```python
from build123d import *

# Parameters (mm, degrees)
SKIZZE1_R                        = 50
SKIZZE1_R_2                      = 20
AUFSATZ_LINEAR_AUSTRAGEN1_DEPTH  = 2.75
F_3_2_3_2_DURCHMESSER_BOHRUNG1_D = 3.2
KREISMUSTER1_COUNT               = 7


with BuildPart() as part:
    # Skizze1 → Aufsatz-Linear austragen1 (new body)
    with BuildSketch(Plane.XY):
        Circle(SKIZZE1_R)
        Circle(SKIZZE1_R_2, mode=Mode.SUBTRACT)
    extrude(amount=AUFSATZ_LINEAR_AUSTRAGEN1_DEPTH)

    # Ø3.2 (3.2) Durchmesser Bohrung1 (through all)
    with Locations(Plane.XY.offset(2.75)):
        with Locations((0, 46)):
            f_3_2_3_2_durchmesser_bohrung1 = Hole(F_3_2_3_2_DURCHMESSER_BOHRUNG1_D / 2)

    # Kreismuster1: Ø3.2 (3.2) Durchmesser Bohrung1 ×7 about axis
    kreismuster1_axis = Axis((0, 0, 0), (0, 0, 1))
    for i in range(1, KREISMUSTER1_COUNT):
        add(f_3_2_3_2_durchmesser_bohrung1.rotate(kreismuster1_axis, i * 360 / KREISMUSTER1_COUNT), mode=Mode.SUBTRACT)


solid = part.part
```
Check sheet for the modelled part. Datum: model origin and axes. Units: mm. Give positions to 0.01 mm unless a question says otherwise; leave off trailing zeros. Write each loop counter-clockwise with the first axis right and the second up, starting at its lowest first coordinate (ties: lowest second). Pieces come first, ordered by that corner, then holes. Notation, with made-up numbers: (17.5, 37.25) - (42.5, 37.25) arc R13 cw to (42.5, 55.25) - close; hole circle Ø9 at (19, 5). An arc over 180 degrees is marked (long way). Answer as a JSON object with one key per item and string values. Group by question number.
1) Sectioned sample at B-B (y = 0). Record the cut outline in (x, z).
2) Thickness scan on probe 1 along X at (y, z) = (-11.5, 1.75); probe 2 along Y at (x, z) = (-21, 0.2); probe 3 along Y at (x, z) = (-18, 1.45). Record the ranges inside material, lowest first. Write a range as from..to.
3) Sectioned sample at D-D (y = 46). Record the cut outline in (x, z), then the cut area to 3 significant figures.
4) Sectioned sample at A-A (x = 0). Record the cut outline in (y, z).
5) Depth check by flat-ended pin: P1, Ø24, axis at x = 0, y = 0, coming from the +Z side. Enter the tip coordinate at first touch or a pass-through.
6) Release check for a two-part mould opening along Y. For faces 1 (the face through (-1, -22, 0)), 2 (the face through (21.319, -42.287, 1.356)), 3 (the face through (47.69, 15.02, 1.36)) record: pulls with the +Y half, pulls with the -Y half, needs draft (parallel to the pull), parting line crosses it, or undercut.
7) Sectioned sample at C-C (z = 1). Give the number of separate pieces and of enclosed holes in the cut face, then the cut area to 3 significant figures.
Geometry results:
{
 "1": {"outline": "(-50, 0) - (-20, 0) - (-20, 2.75) - (-50, 2.75) - close; (20, 0) - (50, 0) - (50, 2.75) - (20, 2.75) - close"},
 "2": {"probe 1": "x = -48.66..-45.83, -43.87..-16.36, 16.36..43.87, 45.83..48.66", "probe 2": "y = -45.38..-42.66, -40.23..45.38", "probe 3": "y = -46.65..-8.72, 8.72..46.65"},
 "3": {"outline": "(-19.6, 0) - (-1.6, 0) - (-1.6, 2.75) - (-19.6, 2.75) - close; (1.6, 0) - (19.6, 0) - (19.6, 2.75) - (1.6, 2.75) - close", "area": "99.0 mm^2"},
 "4": {"outline": "(-50, 0) - (-20, 0) - (-20, 2.75) - (-50, 2.75) - close; (20, 0) - (44.4, 0) - (44.4, 2.75) - (20, 2.75) - close; (47.6, 0) - (50, 0) - (50, 2.75) - (47.6, 2.75) - close"},
 "5": {"P1": "passes through"},
 "6": {"face 1": "needs draft", "face 2": "undercut", "face 3": "parting line crosses it"},
 "7": {"separate pieces": "1", "enclosed holes": "8", "area": "6,540 mm^2"}
}
